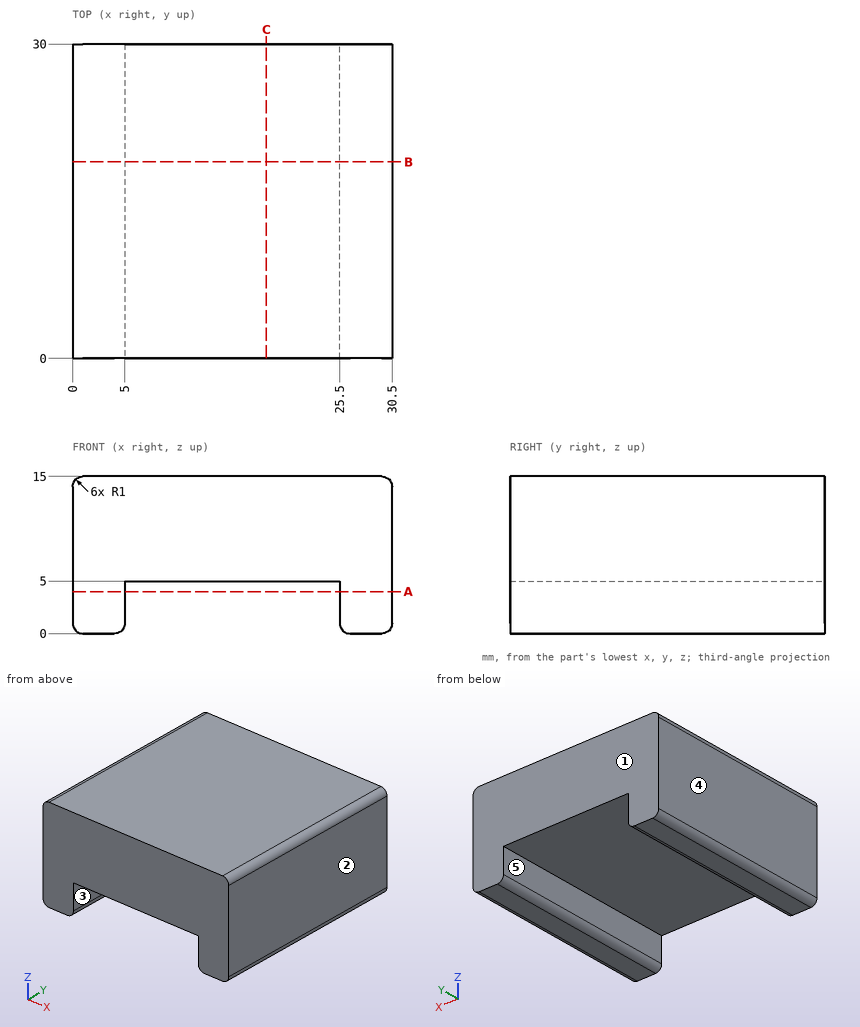
Could you check a few things on this drawing? It's one solid part, dimensions in mm from its lowest x, y, z. A direction names the side the tool comes from. Coordinates: 2 decimals unless noted, no trailing zeros. Order: outer loops, then holes, each group sorted by start corner. A loop starts at its lowest first (then second) coordinate and runs counter-clockwise, first axis right, second up. Notation, with made-up numbers: M 44.5,85 L 94.5,85 A9 cw 94.5,101 Z; hole C 71,-29 d11. An arc over 180 degrees is marked long. Use one line per item in the form item = value. Start each with the question number.
1. Suppose I cut it at C-C on x = 18.5. Write out the boundary of the cut face in (y, z).
2. Suppose I cut it at A-A on z = 4. Write out the boundary of the cut face in (x, y), then the cut area to 3 significant figures.
3. On a 3-axis mill with a long thin cutter (end or side, diameter ignored), from which of +Z, -Z, +X, -X, +Y, -Y can I reach the whole of each face in a straight line? I mean the marked faces 4 and 5. Say none if no direction works.
4. Suppose I cut it at B-B on y = 18.75. Write out the boundary of the cut face in (x, z), then the cut area to 3 significant figures.
5. Please list where these lines run through material, in increasing order: line 1 (X direction, y = 18.25, z = 4.5); line 2 (Z direction, x = 16, y = 15.75).
6. For pin 1 (2 mm diameter, centred on y = 21.5, z = 5.5, fed in from -X); pin 2 (1.5 mm diameter, centred on x = 19.5, z = 3.5, fed in from +Y); pin 3 (8 mm diameter, centred on x = 15.5, y = 23.5, fed in from -Z), each with a flat end and sliding along its axis, tell me the tip position at first contact or that it passes through.
7. We'd pull the mould along X, two halves only. Please class the marked faces 1, 2 and 3: +X half, -X half, draft (parallel to the pull), parting line (faces both ways), or undercut.
Geometry says:
q1.outline = M 0,5 L 30,5 L 30,15 L 0,15 Z
q2.outline = M 0,0 L 5,0 L 5,30 L 0,30 Z; M 25.5,0 L 30.5,0 L 30.5,30 L 25.5,30 Z
q2.area = 300 mm^2
q3.face_4 = +Z, -Z, -X, +Y, -Y
q3.face_5 = -Z, +Y, -Y
q4.outline = M 0,1 A1 ccw 1,0 L 4,0 A1 ccw 5,1 L 5,5 L 25.5,5 L 25.5,1 A1 ccw 26.5,0 L 29.5,0 A1 ccw 30.5,1 L 30.5,14 A1 ccw 29.5,15 L 1,15 A1 ccw 0,14 Z
q4.area = 354 mm^2
q5.line_1 = 0 to 5, 25.5 to 30.5
q5.line_2 = 5 to 15
q6.pin_1 = 0
q6.pin_2 = through
q6.pin_3 = 5
q7.face_1 = draft
q7.face_2 = +X half
q7.face_3 = undercut
